Autodesk Inventor part; units mm, degrees
ref_plane "YZ Plane" through (0, 0, 0) normal (1, 0, 0) x (0, 1, 0)
ref_plane "XZ Plane" through (0, 0, 0) normal (0, 1, 0) x (-1, 0, 0)
ref_plane "XY Plane" through (0, 0, 0) normal (0, 0, 1) x (1, 0, 0)
sketch "Sketch1" plane through (0, 0, 0) normal (0, 1, 0) x (-1, 0, 0)
  arc A0 (6.2517, -1.1129) -> (-6.2517, -1.1129) centre (0, 0) ccw
  arc A1 (-4.1261, -13.0535) -> (4.1261, -13.0535) centre (0, -12.319) ccw
  line L0 (6.2517, -1.1129) -> (4.1261, -13.0535)
  line L1 (-6.2517, -1.1129) -> (-4.1261, -13.0535)
  dimension "d0" = 22.86
  dimension "d1" = 12.7
  dimension "d2" = 8.382
extrude "Extrusion1" add sketch "Sketch1" along normal blind 3.175
sketch "Sketch2" plane through (0, 3.175, 0) normal (0, 1, 0) x (1, 0, 0)
  arc A0 (-6.2517, 1.1129) -> (6.2517, 1.1129) centre (0, 0) ccw
  arc A1 (4.1261, 13.0535) -> (-4.1261, 13.0535) centre (0, 12.319) ccw
hole "Hole1" at (0, 3.175, 0) at (0, 3.175, -12.319) direction (0, -1, 0) diameter 3.683 end through all
properties part number "GripperServoHorn"
CAD build for the part. Positions are in the model's coordinates, mm. Give positions to 0.01 mm unless a question says otherwise; leave off trailing zeros. Loops run counter-clockwise (first coordinate to the right, second up) from the corner with the lowest first, then second, coordinate; pieces in that order, holes last. Notation, with made-up numbers: M 65,57 L 72,57 A29 cw 72,78 Z; hole C 14.25,71 d1. An arc over 180 degrees is marked long. Use one line per item in the form item = value.
Item 1: Slice it at B-B (x = 0). List the corners of the cut face in (y, z) (1 decimal).
Determined:
outline = M 0,-16.5 L 3.2,-16.5 L 3.2,-14.2 L 0,-14.2 Z; M 0,-10.5 L 3.2,-10.5 L 3.2,-1.8 L 0,-1.8 Z; M 0,1.8 L 3.2,1.8 L 3.2,6.3 L 0,6.3 Z
Item 2: Two-plate mould, pull along Z, no slides. Class faces 1 (the face through (0, 0, -5)), 2 (the face through (5.204, 1.565, -7)), 3 (the face through (1.634, 1.565, 0.85)): pulls with the +Z half, pulls with the -Z half, needs draft (parallel to the pull), parting line crosses it, or undercut.
Determined:
face_1 = needs draft
face_2 = pulls with the -Z half
face_3 = undercut
Item 3: Slice it at A-A (z = 0). List the corners of the cut face in (x, y) (1 decimal).
Determined:
outline = M -6.3,0 L -1.8,0 L -1.8,3.2 L -6.3,3.2 Z; M 1.8,0 L 6.3,0 L 6.3,3.2 L 1.8,3.2 Z
Item 4: Slice it at D-D (z = -7.75). List the corners of the cut face in (x, y) (3 decimals).
Determined:
outline = M -5.07,0 L 5.07,0 L 5.07,3.175 L -5.07,3.175 Z
Item 5: Slice it at C-C (y = 2.45). List the corners of the cut face in (x, z), plus the area to 3 significant figures.
Determined:
outline = M -6.25,-1.11 L -4.13,-13.05 A4.19 ccw 4.13,-13.05 L 6.25,-1.11 A6.35 ccw long Z; hole C 0,-12.32 d3.68; hole C 0,0 d3.68
area = 201 mm2
Item 6: Drill centre lines: probe 1 along Z at (x, y) = (0, 1.5); probe 2 along X at (y, z) = (0.8, 0); probe 3 along Z at (x, y) = (-1.25, 1.6). Where is each one in solid material? Low to high. Write a range as from..to.
Determined:
probe_1 = -16.51..-14.16, -10.48..-1.84, 1.84..6.35
probe_2 = -6.35..-1.84, 1.84..6.35
probe_3 = -16.32..-13.67, -10.97..-1.35, 1.35..6.23
Item 7: Flat gauge pin, fed straight in: pin 1 (1 mm diameter, centred on y = 2, z = -6.5, fed in from -X). Where does the tip first touch, or does it go through?
Determined:
pin_1 = -5.38
